```python
from build123d import *

# Parameters (mm, degrees)
F1_DEPTH = 300
F2_R     = 2.49999


# Not quite as in the source:
# - a fillet or chamfer is up to 0.001 mm smaller than in the source, because OpenCascade refuses the exact size


with BuildPart() as f1:
    # F0 (on Right) → F1 (new body)
    with BuildSketch(Plane.YZ):
        with BuildLine():
            Line((0, -10), (0, 0))
            Line((0, 0), (-60, 0))
            ThreePointArc((-60, 0), (-88.2842712475, -11.7157287525), (-100, -40))
            ThreePointArc((-100, -40), (-89.7487373415, -64.7487373415), (-65, -75))
            Line((-65, -75), (-20, -75))
            ThreePointArc((-20, -75), (-5.8578643763, -69.1421356237), (0, -55))
            Line((0, -55), (0, -30))
            Line((0, -30), (-5, -30))
            Line((-5, -30), (-5, -55))
            ThreePointArc((-5, -55), (-7.9289321881, -62.0710678119), (-15, -65))
            Line((-15, -65), (-65, -65))
            ThreePointArc((-65, -65), (-75.6066017178, -60.6066017178), (-80, -50))
            Line((-80, -50), (-80, -30))
            ThreePointArc((-80, -30), (-74.1421356237, -15.8578643763), (-60, -10))
            Line((-60, -10), (0, -10))
        make_face()
    extrude(amount=F1_DEPTH)

    # F2 (radius 2.5 in the source; OpenCascade refuses exactly that, so slightly less here)
    f2_edges = [f1.edges().sort_by_distance(p)[0] for p in [
        (150, 0, -10),
        (150, 0, -30),
        (150, -5, -30),
    ]]
    fillet(f2_edges, radius=F2_R)


solid = f1.part
```
Part model, mm, in its own coordinate system. A direction names the side the tool comes from. Coordinates: 2 decimals unless noted, no trailing zeros. Write each loop counter-clockwise with the first axis right and the second up, starting at its lowest first coordinate (ties: lowest second). Pieces come first, ordered by that corner, then holes.
Item 1: Probe line 1 (Z direction, x = 258.5, y = -23.5); line 2 (Z direction, x = 186.5, y = -13) (3 decimals); line 3 (Y direction, x = 36, z = -54.5). List the from-to ranges inside material, lowest first.
Item 2: Mould opens along Y. For faces 4 (the face through (300, -84, -40)), 5 (the face through (148, 0, -44)), 6 (the face through (148, -80, -40)) say: released by +Y, released by -Y, zero draft, split by the parting line, or undercut.
Item 3: Pin check, flat tips, straight feed: pin 1 (1.5 mm diameter, centred on y = -79.5, z = -49.5, fed in from +X); pin 2 (1 mm diameter, centred on x = 70, z = -15, fed in from -Y); pin 3 (10 mm diameter, centred on x = 232.5, z = -20.5, fed in from -Y); pin 4 (7 mm diameter, centred on x = 145, z = -47, fed in from -Y). Stop position of each tip, or through.
Item 4: Slice it at B-B (z = -61). Write the cut outline in (x, y).
Item 5: Which spindle directions (+Z, -Z, +X, -X, +Y, -Y) get a long thin tool onto all of the face, cutting with end or side? Do faces 1 (the face through (147.9, -75.49, -60.72)), 2 (the face through (148, -32, -10)), 3 (the face through (147.9, -87.972, -11.406)). Say none if no direction does.
Item 6: Slice it at D-D (z = -24). Write the cut outline in (x, y), and give its area (3 significant figures).
Item 7: Slice it at A-A (y = -28.5). Write the cut outline in (x, z).
Results found:
1. line 1: z = -75 to -65, -10 to 0
1. line 2: z = -73.735 to -64.798, -10 to 0
1. line 3: y = -96.86 to -79.31, -5 to 0
2. face 4: zero draft
2. face 5: released by +Y
2. face 6: undercut
3. pin 1: stops at x = 300
3. pin 2: stops at y = -91.62
3. pin 3: stops at y = -97.28
3. pin 4: stops at y = -99.82
4. outline: (0, -93) - (300, -93) - (300, -75.2) - (0, -75.2) - close; (0, -7) - (300, -7) - (300, -0.92) - (0, -0.92) - close
5. face 1: +X, -X
5. face 2: +X, -X, +Y
5. face 3: +Z, +X, -X, -Y
6. outline: (0, -96.66) - (300, -96.66) - (300, -79.08) - (0, -79.08) - close
6. area: 5,270 mm2
7. outline: (0, -75) - (300, -75) - (300, -65) - (0, -65) - close; (0, -10) - (300, -10) - (300, 0) - (0, 0) - close
